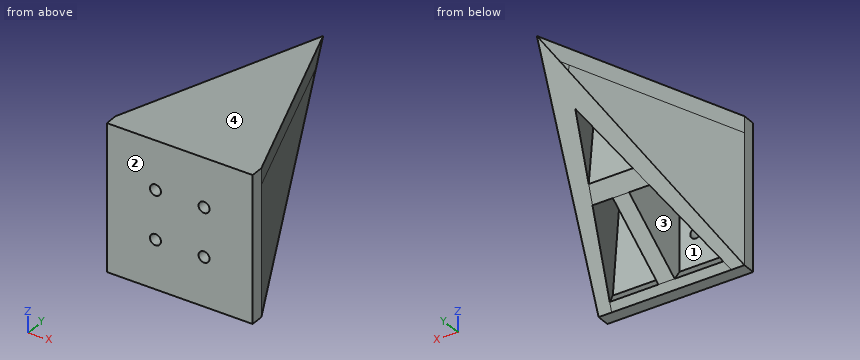
```python
from build123d import *

# Parameters (mm, degrees)
SKETCH_1_W          = 45
SKETCH_1_H          = 45
SKETCH_1_R          = 1.7
EXTRUDE_1_DEPTH     = 4
EXTRUDE_2_DEPTH     = 5
EXTRUDE_3_DEPTH     = 65.785596942
EXTRUDE_4_DEPTH     = 65.785596942
CUT_EXTRUDE_1_DEPTH = 92.553486945
CUT_EXTRUDE_2_DEPTH = 85.512691631
EXTRUDE_9_REACH     = 86.713
CHAMFER_1_SIZE      = 5
EXTRUDE_10_REACH    = 86.713
EXTRUDE_11_REACH    = 88.671
SKETCH_13_W         = 5
SKETCH_13_H         = 28.755225939


with BuildPart() as part:
    # 草图1 → 凸台-拉伸1 (new body)
    with BuildSketch(Plane(origin=(0, 0, 0), x_dir=(1, 0, 0), z_dir=(0, 1, 0))):
        with Locations((22.5, 22.5)):
            Rectangle(SKETCH_1_W, SKETCH_1_H)
        with Locations(Location((15, 30, 0), (0, 0, 270))):
            Circle(SKETCH_1_R, mode=Mode.SUBTRACT)
        with Locations(Location((30, 30, 0), (0, 0, 270))):
            Circle(SKETCH_1_R, mode=Mode.SUBTRACT)
        with Locations(Location((15, 15, 0), (0, 0, 270))):
            Circle(SKETCH_1_R, mode=Mode.SUBTRACT)
        with Locations(Location((30, 15, 0), (0, 0, 270))):
            Circle(SKETCH_1_R, mode=Mode.SUBTRACT)
    extrude(amount=EXTRUDE_1_DEPTH)

    # 草图2 → 凸台-拉伸2 (add)
    with BuildSketch(Plane.XY):
        Polygon((0, 4), (22.5, 65.818241938), (45, 4), align=None)
    extrude(amount=-EXTRUDE_2_DEPTH)

    # 草图3 → 凸台-拉伸3 (add, along a direction that is not the sketch's normal)
    with BuildSketch(Plane(origin=(0, 4, 0), x_dir=(1, 0, 0), z_dir=(0, 1, 0))):
        Polygon((0, 5), (0, 45), (4, 45), (7, 5), align=None)
    extrude(amount=EXTRUDE_3_DEPTH, dir=(0.34202014332566566, 0.9396926207859095, 0))

    # 草图4 → 凸台-拉伸4 (add, along a direction that is not the sketch's normal)
    with BuildSketch(Plane(origin=(0, 4, 0), x_dir=(1, 0, 0), z_dir=(0, 1, 0))):
        Polygon((45, 45), (41, 45), (38, 5), (45, 5), align=None)
    extrude(amount=EXTRUDE_4_DEPTH, dir=(-0.3420201433256661, 0.9396926207859094, 0))

    # 草图5 → 切除-拉伸1 (cut, through all)
    with BuildSketch(Plane.XY):
        Polygon((22.5, 65.818241938), (19, 56.20207097), (11, 56.20207097), (11, 66.20207097), (34, 66.20207097), (34, 56.20207097), (26, 56.20207097), align=None)
    extrude(amount=-CUT_EXTRUDE_1_DEPTH, mode=Mode.SUBTRACT)

    # 草图6 → 切除-拉伸2 (cut, through all, along a direction that is not the sketch's normal)
    with BuildSketch(Plane(origin=(41.02157519, 14.930632332, 0), x_dir=(0, 0, -1), z_dir=(0.9396926207859093, 0.3420201433256662, 0))):
        Polygon((0, 54.153463037), (45, -11.632135967), (45, 54.153463037), align=None)
    extrude(amount=-CUT_EXTRUDE_2_DEPTH, dir=(1, 0, 0), mode=Mode.SUBTRACT)

    # 凸台-拉伸9: up to this plane
    extrude_9_end = Plane(origin=(26.5, 65.818241938, -45), z_dir=(-0.9373675520499937, 0.34117388751316935, 0.07030256640374952))
    # 草图8 → 凸台-拉伸9 (add, up to the surface)
    with BuildSketch(Plane(origin=(34.338725854, 12.498274094, 2.575404439), x_dir=(-0.06606280287191471, -0.024044893837572568, 0.9975257135317598), z_dir=(-0.9373675520499937, -0.34117388751316985, -0.07030256640374943)), mode=Mode.PRIVATE) as extrude_9_sk1:
        Polygon((-47.693411602, -10.264055393), (-46.016852855, -7.776255006), (-42.693411602, -10.136115185), align=None)
    extrude_9_tool1 = split(extrude(extrude_9_sk1.sketch, amount=EXTRUDE_9_REACH, dir=(-1, 0, 0), mode=Mode.PRIVATE), bisect_by=extrude_9_end, keep=Keep.BOTH, mode=Mode.PRIVATE)
    add(extrude_9_tool1.solids().sort_by_distance((40.554764, 4.765818, -42.779987))[0])

    # 倒角1
    chamfer_1_edges = [part.edges().sort_by_distance(p)[0] for p in [
        (22.5, 4, -5),
    ]]
    chamfer(chamfer_1_edges, length=CHAMFER_1_SIZE)

    # 凸台-拉伸10: up to this plane
    extrude_10_end = Plane(origin=(26.5, 65.818241938, -45), z_dir=(-0.9373675520499937, 0.34117388751316935, 0.07030256640374952))
    # 草图10 → 凸台-拉伸10 (add, up to the surface)
    with BuildSketch(Plane(origin=(34.338725854, 12.498274094, 2.575404439), x_dir=(-0.06606280287191474, -0.024044893837572537, 0.9975257135317598), z_dir=(-0.9373675520499936, -0.34117388751316985, -0.07030256640374943)), mode=Mode.PRIVATE) as extrude_10_sk1:
        Polygon((-27.358712809, 19.91005667), (-30.728273238, 14.91005667), (-7.594194652, 14.91005667), (-7.594194652, 19.91005667), align=None)
    extrude_10_tool1 = split(extrude(extrude_10_sk1.sketch, amount=EXTRUDE_10_REACH, dir=(-1, 0, 0), mode=Mode.PRIVATE), bisect_by=extrude_10_end, keep=Keep.BOTH, mode=Mode.PRIVATE)
    add(extrude_10_tool1.solids().sort_by_distance((29.618174, 29.237872, -15.720115))[0])

    # 凸台-拉伸11: up to this plane
    extrude_11_end = Plane(origin=(0, 0, -5), z_dir=(0, 0, -1))
    # 草图13 → 凸台-拉伸11 (add, up to the surface)
    with BuildSketch(Plane(origin=(0, 22.796896106, -31.316978642), x_dir=(-1, 0, 0), z_dir=(0, 0.5885247359201023, -0.8084792113654956)), mode=Mode.PRIVATE) as extrude_11_sk1:
        with Locations((-22.5, -8.872083302)):
            Rectangle(SKETCH_13_W, SKETCH_13_H)
    extrude_11_tool1 = split(extrude(extrude_11_sk1.sketch, amount=EXTRUDE_11_REACH, dir=(0, 0, 1), mode=Mode.PRIVATE), bisect_by=extrude_11_end, keep=Keep.BOTH, mode=Mode.PRIVATE)
    add(extrude_11_tool1.solids().sort_by_distance((22.5, 15.624001, -36.538419))[0])


solid = part.part
```
Part model, mm, in its own coordinate system. Face numbers are marked on the shaded views. A direction names the side the tool comes from. Round coordinates to 2 decimals unless told otherwise and drop trailing zeros. Loops run counter-clockwise (first coordinate to the right, second up) from the corner with the lowest first, then second, coordinate; pieces in that order, holes last.
Item 1: Mould opens along X. For the marked faces 3 and 4 say: +X half, -X half, draft (parallel to the pull), parting line (faces both ways), or undercut.
Item 2: Drill centre lines: line 1 (X direction, y = 2, z = -15); line 2 (Y direction, x = 33.5, z = -38.5); line 3 (X direction, y = 15, z = -19). Where is each one in solid material? Low to high.
Item 3: Cut at B-B, the plane x = 24. Give the cut face in (y, z).
Item 4: Cut at A-A, the plane z = -20. Give the cut face in (x, y) (3 decimals), then the cut area to 3 significant figures.
Item 5: Drop flat-ended pins along their axis: P1, Ø5, axis at x = 31.5, y = 10, coming from the +Z side; P2, Ø10, axis at y = 13, z = -25, coming from the +X side; P3, Ø12.5, axis at x = 13.5, z = -28, coming from the +Y side; P4, Ø8, axis at x = 21, y = 27.5, coming from the -Z side. Give the stop position or say it passes through.
Item 6: 3-axis set-ups, long thin cutter, end or side, ignore diameter. For the marked faces 1 and 2: which of +Z, -Z, +X, -X, +Y, -Y reach the whole face in a straight line?
Item 7: Cut at D-D, the plane y = 43.5. Give the cut face in (x, z), then the cut area to 3 significant figures.
Item 8: Cut at C-C, the plane z = -30. Give the cut face in (x, y) (3 decimals), then the cut area to 3 significant figures.
A:
1. face 3: undercut
1. face 4: draft
2. line 1: x = 0 to 13.3, 16.7 to 28.3, 31.7 to 45
2. line 2: y = 0 to 4
2. line 3: x = 4 to 9.95, 20 to 25, 35.05 to 41
3. outline: (0, -45) - (4, -45) - (31.87, -24.72) - (31.39, -5) - (42.46, -5) - (44.61, -15.43) - (61.7, -3) - (61.7, 0) - (0, 0) - close
4. outline: (0, 0) - (45, 0) - (45, 4) - (32.5, 38.343) - (26.625, 38.343) - (29.024, 31.752) - (15.976, 31.752) - (18.375, 38.343) - (12.5, 38.343) - (0, 4) - close; hole (5.875, 4) - (20, 4) - (20, 27.053) - (14.266, 27.053) - close; hole (25, 4) - (39.125, 4) - (30.734, 27.053) - (25, 27.053) - close
4. area: 768 mm2
5. P1: stops at z = 0
5. P2: stops at x = 43.54
5. P3: stops at y = 35.94
5. P4: stops at z = -30.81
6. face 1: none
6. face 2: +Z, -Z, +X, -X, -Y
7. outline: (14.38, -16.25) - (20.53, -16.25) - (21.38, -5) - (23.62, -5) - (24.47, -16.25) - (30.62, -16.25) - (30.62, 0) - (14.38, 0) - close
7. area: 229 mm2
8. outline: (0, 0) - (13.3, 0) - (13.3, 4) - (5.125, 4) - (12.625, 24.606) - (7.5, 24.606) - (0, 4) - close; (16.7, 0) - (28.3, 0) - (28.3, 4) - (25, 4) - (25, 24.606) - (20, 24.606) - (20, 4) - (16.7, 4) - close; (31.7, 0) - (45, 0) - (45, 4) - (37.5, 24.606) - (32.375, 24.606) - (39.875, 4) - (31.7, 4) - close
8. area: 467 mm2
